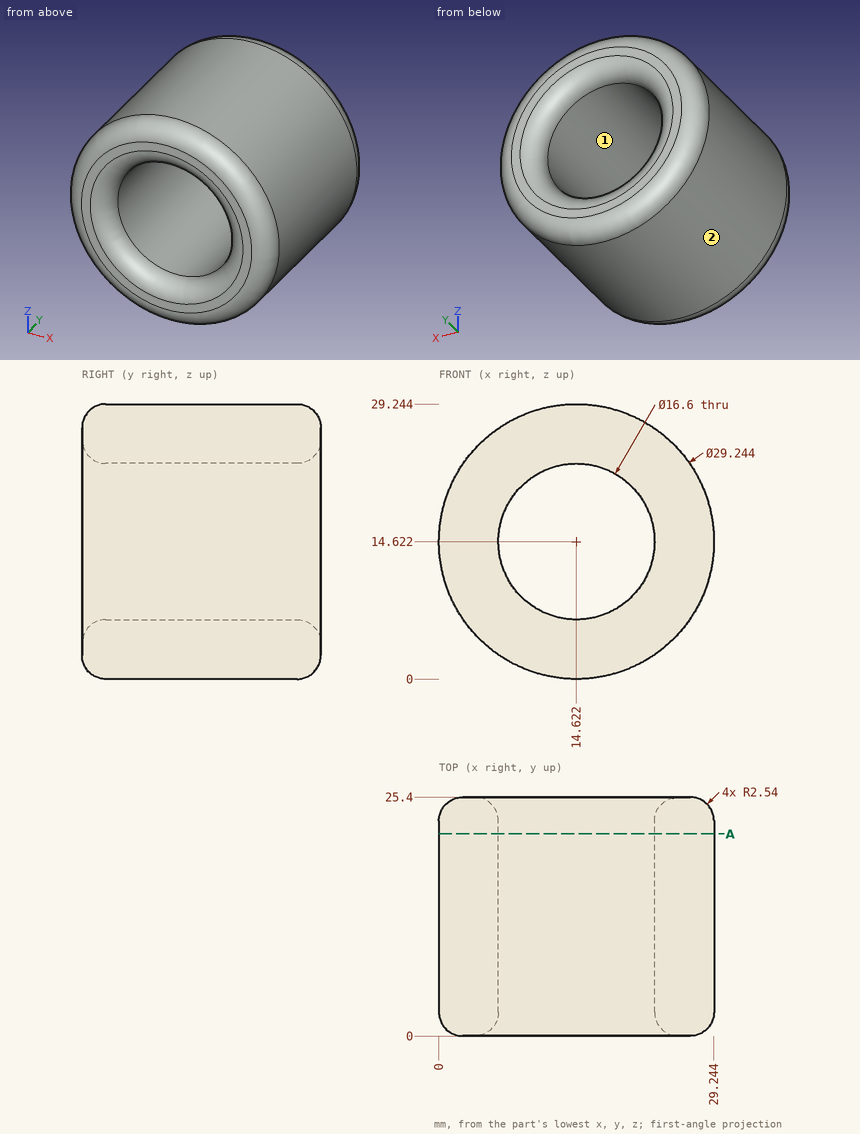
Check sheet for the drawn part. Datum: minimum x, y, z corner. Units: mm. Give positions to 0.01 mm unless a question says otherwise; leave off trailing zeros. Loops run counter-clockwise (first coordinate to the right, second up) from the corner with the lowest first, then second, coordinate; pieces in that order, holes last.
1) Sectioned sample at A-A, the plane y = 21.5. Enter the section's corners in (x, z).
2) Thickness scan on line 1 along Z through (x, y) = (15, 20.5) (1 decimal); line 2 along X through (y, z) = (9, 14.75); line 3 along Z through (x, y) = (19, 24) (1 decimal). Record the ranges inside material, lowest first.
3) Depth check by flat-ended pin: pin 1 Ø1 at (y, z) = (7, 22) entering from +X; pin 2 Ø10 at (y, z) = (12.5, 8) entering from -X; pin 3 Ø10 at (x, y) = (21, 21.5) entering from -Z (3 decimals). Enter the tip coordinate at first touch or a pass-through.
4) Draft check along Z on the marked faces 1 and 2. Enter one of: pulls with the +Z half, pulls with the -Z half, needs draft (parallel to the pull), parting line crosses it, or undercut.
Answers:
1. outline: circle Ø29.24 at (14.62, 14.62); hole circle Ø16.6 at (14.62, 14.62)
2. line 1: z = 0 to 6.3, 22.9 to 29.2
2. line 2: x = 0 to 6.32, 22.92 to 29.24
2. line 3: z = 1 to 7.3, 22 to 28.3
3. pin 1: stops at x = 27.53
3. pin 2: stops at x = 0.09
3. pin 3: stops at z = 0.065
4. face 1: undercut
4. face 2: parting line crosses it
